Geometry check sheet. Reference: the model listing, model coordinates, mm. A direction names the side the tool comes from. Coordinates: 2 decimals unless noted, no trailing zeros. Write each loop counter-clockwise with the first axis right and the second up, starting at its lowest first coordinate (ties: lowest second). Pieces come first, ordered by that corner, then holes. Notation, with made-up numbers: (-26, 56.5) -> (17, 56.5) arc R21 cw to (17, 81.5) -> close; hole circle Ø3 at (-11.75, 44). An arc over 180 degrees is marked (long way). Answer in a Markdown table with one row per item. Add a question column.
1. Set-up check for faces 1 (the flat face through (0, -4, 2.5)), 2 (the flat face through (0.33, 2.807, 1.15)): record each of +Z, -Z, +X, -X, +Y, -Y from which the full face is reachable in a straight line by a thin tool's end or side.
2. Scan lines: L1, parallel to Y at x = 0, z = -1.1 (3 decimals); L2, parallel to Y at x = 0, z = -0.9 (3 decimals); L3, parallel to Z at x = 0, y = 7.75 (3 decimals). Record each from-to range of solid material in increasing order. Write a range as from..to.
3. Cross-section at C-C on z = 0. Give the number of separate pieces and of enclosed holes in the cut face, and give its area (3 significant figures).
4. Cross-section at B-B on y = 3.25. Record the cut outline in (x, z) (3 decimals).
5. Mould release check, pull along X, two halves, no side actions. Record for faces 3 (the cylindrical face through (-1.016, 5.947, 0.133)), 4 (the cylindrical face through (-9, 0, 0)), 5 (the flat face through (0, -4, -2.5)): pulls with the +X half, pulls with the -X half, needs draft (parallel to the pull), parting line crosses it, or undercut.
6. Cross-section at A-A on x = 0. Record the cut outline in (y, z) (3 decimals).
7. Depth check by flat-ended pin: P1, Ø1, axis at y = 3.5, z = -1.5, coming from the -X side; P2, Ø1, axis at y = -1.5, z = 1.5, coming from the -X side; P3, Ø1, axis at y = -6.5, z = 1.5, coming from the -X side. Enter the tip coordinate at first touch or a pass-through.
8. Cross-section at D-D on x = -3. Record the cut outline in (y, z).
```python
from build123d import *

# Parameters (mm, degrees)
SKETCH1_R              = 9
BOSS_EXTRUDE1_DEPTH    = 2.5
M2_5_CLEARANCE_HOLE2_D = 2.5
CIRPATTERN1_COUNT      = 3
SKETCH7_W              = 1.025
SKETCH7_H              = 6.192782739


with BuildPart() as part:
    # Sketch1 → Boss-Extrude1 (new body, symmetric)
    with BuildSketch(Plane.XY):
        Circle(SKETCH1_R)
        with BuildLine():
            Line((-1.5875, 2.807217261), (1.5875, 2.807217261))
            ThreePointArc((1.5875, 2.807217261), (0, -3.225), (-1.5875, 2.807217261))
        make_face(mode=Mode.SUBTRACT)
    extrude(amount=BOSS_EXTRUDE1_DEPTH, both=True)

    # M2.5 Clearance Hole2 (through all)
    with Locations(Plane.XY.offset(2.5)):
        with Locations((0, -6.5)):
            m2_5_clearance_hole2 = Hole(M2_5_CLEARANCE_HOLE2_D / 2)

    # CirPattern1: M2.5 Clearance Hole2 ×3 about axis
    cirpattern1_axis = Axis((0, 0, 0), (0, 0, 1))
    for i in range(1, CIRPATTERN1_COUNT):
        add(m2_5_clearance_hole2.rotate(cirpattern1_axis, i * 360 / CIRPATTERN1_COUNT), mode=Mode.SUBTRACT)

    # Sketch7 → M2.5x0.45 Tapped Hole1 (revolve, cut)
    with BuildSketch(Plane(origin=(0, 2.807217261, 0), x_dir=(0, 0, -1), z_dir=(1, 0, 0))):
        with Locations((0.5125, 3.09639137)):
            Rectangle(SKETCH7_W, SKETCH7_H)
    revolve(axis=Axis((0, -3.542782739, 0), (0, 1, 0)), mode=Mode.SUBTRACT)


solid = part.part
```
Results found:
| question | item | result |
|---|---|---|
| 1 | face 1 | +Z, +X, -X, +Y, -Y |
| 1 | face 2 | +Z, -Z |
| 2 | L1 | y = -9..-7.75, -5.25..-3.225, 2.807..9 |
| 2 | L2 | y = -9..-7.75, -5.25..-3.225 |
| 2 | L3 | z = -2.5..-1.025, 1.025..2.5 |
| 3 | separate pieces | 1 |
| 3 | enclosed holes | 3 |
| 3 | area | 195 mm^2 |
| 4 | outline | (-8.393, -2.5) -> (-6.879, -2.5) -> (-6.879, 2.5) -> (-8.393, 2.5) -> close; (-4.379, -2.5) -> (4.379, -2.5) -> (4.379, 2.5) -> (-4.379, 2.5) -> close; (6.879, -2.5) -> (8.393, -2.5) -> (8.393, 2.5) -> (6.879, 2.5) -> close; hole circle Ø2.05 at (0, 0) |
| 5 | face 3 | undercut |
| 5 | face 4 | parting line crosses it |
| 5 | face 5 | needs draft |
| 6 | outline | (-9, -2.5) -> (-7.75, -2.5) -> (-7.75, 2.5) -> (-9, 2.5) -> close; (-5.25, -2.5) -> (-3.225, -2.5) -> (-3.225, 2.5) -> (-5.25, 2.5) -> close; (2.807, -2.5) -> (9, -2.5) -> (9, -1.025) -> (2.807, -1.025) -> close; (2.807, 1.025) -> (9, 1.025) -> (9, 2.5) -> (2.807, 2.5) -> close |
| 7 | P1 | stops at x = -8.49 |
| 7 | P2 | stops at x = -8.94 |
| 7 | P3 | stops at x = -6.71 |
| 8 | outline | (-8.49, -2.5) -> (-1.18, -2.5) -> (-1.18, 2.5) -> (-8.49, 2.5) -> close; (1.18, -2.5) -> (8.49, -2.5) -> (8.49, 2.5) -> (1.18, 2.5) -> close |
